The figure shows three views and two pictorial views of one solid part (mm, origin at its lowest corner). Answer the questions. Coordinates: 2 decimals unless noted, no trailing zeros. Loops run counter-clockwise (first coordinate to the right, second up) from the corner with the lowest first, then second, coordinate; pieces in that order, holes last. Notation, with made-up numbers: M 38,30 L 89,30 A13 cw 89,51 Z; hole C -0.5,-35 d9. An arc over 180 degrees is marked long. Answer as a JSON object with one key per item and string values. Group by question number.
1. A cutting plane is placed at D-D on y = 1.45. State how many separate pieces and enclosed holes the cut face has, and give its area (3 significant figures).
2. A cutting plane is placed at B-B on z = 145. Give the vertices of the cut face in (x, y) (1 decimal).
3. Straight lines are drawn through the part: L1, parallel to X at y = 0.9, z = 75; L2, parallel to Z at x = 125, y = 2.15 (1 decimal); L3, parallel to X at y = 0.45, z = 88.5 (1 decimal). For each, find the intervals that lie inside material, in ascending order.
4. A cutting plane is placed at A-A on x = 75. Give the vertices of the cut face in (y, z).
5. Given pin 1 (8 mm diameter, centred on x = 25.5, z = 124.5, fed in from +Y), flat-ended and moving along its own axis, determine where the tip first touches the part or whether it passes through.
6. Determine the mould class of the marked faces 1 and 2 for opening direction Y: released by +Y, released by -Y, zero draft, split by the parting line, or undercut.
7. A cutting plane is placed at C-C on x = 145. Give the vertices of the cut face in (y, z) (1 decimal).
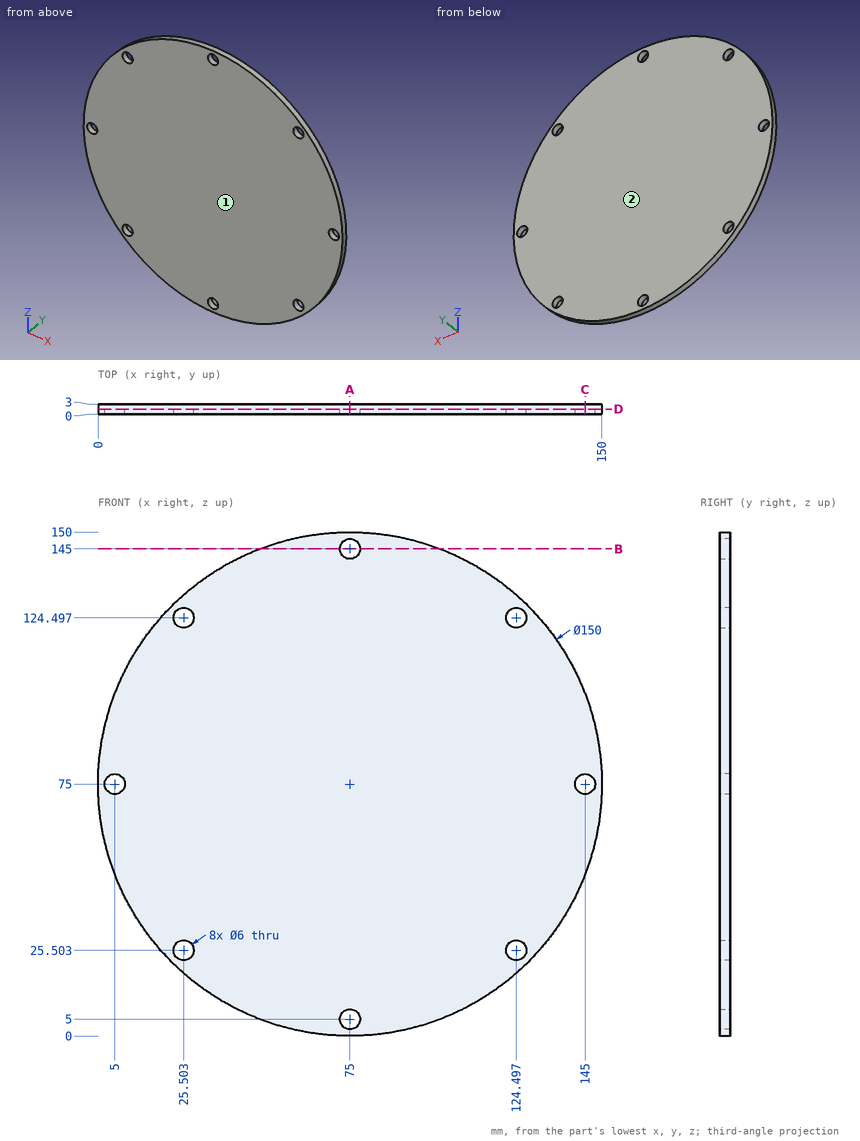
From the geometry:
{
 "1": {"separate pieces": "1", "enclosed holes": "8", "area": "17,400 mm²"},
 "2": {"outline": "M 48.1,0 L 72,0 L 72,3 L 48.1,3 Z; M 78,0 L 101.9,0 L 101.9,3 L 78,3 Z"},
 "3": {"L1": "x = 0 to 2, 8 to 142, 148 to 150", "L2": "z = 19.1 to 22.5, 28.5 to 121.5, 127.5 to 130.9", "L3": "x = 1.2 to 148.8"},
 "4": {"outline": "M 0,0 L 3,0 L 3,2 L 0,2 Z; M 0,8 L 3,8 L 3,142 L 0,142 Z; M 0,148 L 3,148 L 3,150 L 0,150 Z"},
 "5": {"pin 1": "stops at y = 3"},
 "6": {"face 1": "released by -Y", "face 2": "released by +Y"},
 "7": {"outline": "M 0,48.1 L 3,48.1 L 3,72 L 0,72 Z; M 0,78 L 3,78 L 3,101.9 L 0,101.9 Z"}
}
